```python
from build123d import *
from OCP.BRepFilletAPI import BRepFilletAPI_MakeFillet

# Parameters (mm, degrees)
SKETCH_1_W             = 3
SKETCH_1_H             = 12
SKETCH_1_W_2           = 8
SKETCH_1_H_2           = 3
EXTRUDE_1_DEPTH        = 3
SKETCH_3_R             = 1
CUT_EXTRUDE_1_DEPTH    = 55.203320931
SKETCH_4_W             = 1
SKETCH_4_H             = 7
CUT_EXTRUDE_2_DEPTH    = 55.203320931
SKETCH_6_R             = 1.35
CUT_EXTRUDE_3_DEPTH    = 55.203320931
CUT_EXTRUDE_4_DEPTH    = 55.203320931
CUT_EXTRUDE_6_DEPTH    = 55.203320931
FILLET_1_R             = 2
FILLET_2_R1            = 5
FILLET_2_R2            = 1
FILLET_2_R3            = 2
CUT_EXTRUDE_5602_DEPTH = 55.203320931
FILLET_3_R1            = 1
FILLET_3_R2            = 5


with BuildPart() as part:
    # 草图1 → 凸台-拉伸1 (new body)
    with BuildSketch(Plane(origin=(0, 0, 0), x_dir=(1, 0, 0), z_dir=(0, 1, 0))):
        Polygon((15, 26), (15, 52), (0, 52), (-15, 52), (-15, 46), (0, 0), (7, 0), align=None)
        with Locations((3.5, 9)):
            Rectangle(SKETCH_1_W, SKETCH_1_H, mode=Mode.SUBTRACT)
        with Locations((3.5, 33)):
            Rectangle(SKETCH_1_W, SKETCH_1_H, mode=Mode.SUBTRACT)
        with Locations((-8, 47.5)):
            Rectangle(SKETCH_1_W_2, SKETCH_1_H_2, mode=Mode.SUBTRACT)
        with Locations((8, 47.5)):
            Rectangle(SKETCH_1_W_2, SKETCH_1_H_2, mode=Mode.SUBTRACT)
    extrude(amount=EXTRUDE_1_DEPTH)

    # 草图3 → 切除-拉伸1 (cut, through all)
    with BuildSketch(Plane(origin=(0, 3, 0), x_dir=(1, 0, 0), z_dir=(0, 1, 0))):
        with Locations((5, 4)):
            Circle(SKETCH_3_R)
        with Locations((5, 14)):
            Circle(SKETCH_3_R)
        with Locations((2, 4)):
            Circle(SKETCH_3_R)
        with Locations((2, 14)):
            Circle(SKETCH_3_R)
        with Locations((2, 28)):
            Circle(SKETCH_3_R)
        with Locations((2, 38)):
            Circle(SKETCH_3_R)
        with Locations((5, 28)):
            Circle(SKETCH_3_R)
        with Locations((5, 38)):
            Circle(SKETCH_3_R)
        with Locations((-5, 49)):
            Circle(SKETCH_3_R)
        with Locations((-11, 49)):
            Circle(SKETCH_3_R)
        with Locations((-11, 46)):
            Circle(SKETCH_3_R)
        with Locations((-5, 46)):
            Circle(SKETCH_3_R)
        with Locations((5, 46)):
            Circle(SKETCH_3_R)
        with Locations((11, 46)):
            Circle(SKETCH_3_R)
        with Locations((11, 49)):
            Circle(SKETCH_3_R)
        with Locations((5, 49)):
            Circle(SKETCH_3_R)
    extrude(amount=-CUT_EXTRUDE_1_DEPTH, mode=Mode.SUBTRACT)

    # 草图4 → 切除-拉伸2 (cut, through all)
    with BuildSketch(Plane.XZ):
        with Locations((14.5, -48.5)):
            Rectangle(SKETCH_4_W, SKETCH_4_H)
    extrude(amount=-CUT_EXTRUDE_2_DEPTH, mode=Mode.SUBTRACT)

    # 草图6 → 切除-拉伸3 (cut, through all)
    with BuildSketch(Plane(origin=(0, 3, 0), x_dir=(1, 0, 0), z_dir=(0, 1, 0))):
        with Locations(Location((10, 31, 0), (0, 0, 270))):
            Circle(SKETCH_6_R)
        with Locations(Location((10, 41, 0), (0, 0, 90))):
            Circle(SKETCH_6_R)
    extrude(amount=-CUT_EXTRUDE_3_DEPTH, mode=Mode.SUBTRACT)

    # 草图7 → 切除-拉伸4 (cut, through all)
    with BuildSketch(Plane(origin=(0, 3, 0), x_dir=(1, 0, 0), z_dir=(0, 1, 0))):
        Polygon((-2, 15.810109656), (-10.540181634, 42), (-2, 42), align=None)
    extrude(amount=-CUT_EXTRUDE_4_DEPTH, mode=Mode.SUBTRACT)

    # 草图9 → 切除-拉伸6 (cut, through all)
    with BuildSketch(Plane.XZ):
        Polygon((11.923076923, -16), (9.5, -16), (9.5, -8.125), align=None)
    extrude(amount=-CUT_EXTRUDE_6_DEPTH, mode=Mode.SUBTRACT)

    # 圆角1
    # the kernel refuses this fillet: 2 mm, written as the material it takes off along each edge
    with BuildSketch(Plane(origin=(15, -4.330127019, -45), x_dir=(0, 0, 1), z_dir=(0, 1, 0))) as fillet_1_piece_1:
        with BuildLine():
            CenterArc((1.732050808, -2), FILLET_1_R, 90, 60)
            Line((0, -1), (-0.034641016, -0.98))
            ThreePointArc((-0.034641016, -0.98), (-0.04, -0.5), (-0.04, 0))
            Line((-0.04, 0), (0, 0.04))
            Line((0, 0.04), (1.732050808, 0.04))
            Line((1.732050808, 0.04), (1.732050808, 0))
        make_face()
    extrude(amount=11.660254038, mode=Mode.SUBTRACT)
    with BuildSketch(Plane(origin=(7, -3.692873273, 0), x_dir=(-1, 0, 0), z_dir=(0, 1, 0))) as fillet_1_piece_2:
        with BuildLine():
            CenterArc((FILLET_1_R * 0.738574654518, -FILLET_1_R), FILLET_1_R, 90, 72.897271031)
            Line((-FILLET_1_R * 0.217204354204, -FILLET_1_R * 0.705914151162), (-FILLET_1_R * 0.236319934378, -FILLET_1_R * 0.700032434186))
            Line((-FILLET_1_R * 0.236319934378, -FILLET_1_R * 0.700032434186), (-FILLET_1_R * 0.0147714930904, FILLET_1_R * 0.02))
            Line((-FILLET_1_R * 0.0147714930904, FILLET_1_R * 0.02), (FILLET_1_R * 0.738574654518, FILLET_1_R * 0.02))
            Line((FILLET_1_R * 0.738574654518, FILLET_1_R * 0.02), (FILLET_1_R * 0.738574654518, 0))
        make_face()
    extrude(amount=10.385746545, mode=Mode.SUBTRACT)
    with BuildSketch(Plane(origin=(0, -3.628682784, 0), x_dir=(1, 0, 0), z_dir=(0, 1, 0))) as fillet_1_piece_3:
        with BuildLine():
            CenterArc((FILLET_1_R * 0.725736556818, FILLET_1_R), FILLET_1_R, 198.060471936, 71.939528064)
            Line((-FILLET_1_R * 0.224993282664, FILLET_1_R * 0.689979400169), (-FILLET_1_R * 0.244007879453, FILLET_1_R * 0.683778988172))
            Line((-FILLET_1_R * 0.244007879453, FILLET_1_R * 0.683778988172), (-FILLET_1_R * 0.0145147311364, -FILLET_1_R * 0.02))
            Line((-FILLET_1_R * 0.0145147311364, -FILLET_1_R * 0.02), (FILLET_1_R * 0.725736556818, -FILLET_1_R * 0.02))
            Line((FILLET_1_R * 0.725736556818, -FILLET_1_R * 0.02), (FILLET_1_R * 0.725736556818, 0))
        make_face()
    extrude(amount=10.257365568, mode=Mode.SUBTRACT)
    with BuildSketch(Plane(origin=(-15, -0.794627205, -46), x_dir=(0.31002059983091895, 0, 0.9507298394814782), z_dir=(0, 1, 0))) as fillet_1_piece_4:
        with BuildLine():
            CenterArc((FILLET_1_R * 0.158925440907, FILLET_1_R), FILLET_1_R, 251.939528064, 18.060471936)
            Line((-FILLET_1_R * 0.151095158923, FILLET_1_R * 0.0492701605185), (-FILLET_1_R * 0.15729557092, FILLET_1_R * 0.0302555637289))
            Line((-FILLET_1_R * 0.15729557092, FILLET_1_R * 0.0302555637289), (-FILLET_1_R * 0.00317850881815, -FILLET_1_R * 0.02))
            Line((-FILLET_1_R * 0.00317850881815, -FILLET_1_R * 0.02), (FILLET_1_R * 0.158925440907, -FILLET_1_R * 0.02))
            Line((FILLET_1_R * 0.158925440907, -FILLET_1_R * 0.02), (FILLET_1_R * 0.158925440907, 0))
        make_face()
    extrude(amount=4.589254409, mode=Mode.SUBTRACT)
    with BuildSketch(Plane(origin=(14, -5, -52), x_dir=(-1, 0, 0), z_dir=(0, 1, 0)), Plane(origin=(-15, -5, -52), x_dir=(0, 0, 1), z_dir=(0, 1, 0))) as fillet_1_piece_5:
        with BuildLine():
            CenterArc((FILLET_1_R, FILLET_1_R), FILLET_1_R, 180, 90)
            Line((0, FILLET_1_R), (-FILLET_1_R * 0.02, FILLET_1_R))
            Line((-FILLET_1_R * 0.02, FILLET_1_R), (-FILLET_1_R * 0.02, -FILLET_1_R * 0.02))
            Line((-FILLET_1_R * 0.02, -FILLET_1_R * 0.02), (FILLET_1_R, -FILLET_1_R * 0.02))
            Line((FILLET_1_R, -FILLET_1_R * 0.02), (FILLET_1_R, 0))
        make_face()
    extrude(amount=13, mode=Mode.SUBTRACT)

    # 圆角2: one fillet with a radius per group of edges: ONE call of the kernel's fillet builder (fillet() takes one radius for all edges)
    fillet_2_edges_1 = [part.edges().sort_by_distance(p)[0] for p in [
        (15, 1.5, -26),
    ]]
    fillet_2_edges_2 = [part.edges().sort_by_distance(p)[0] for p in [
        (-10.540181634, 1.5, -42),
        (-2, 1.5, -42),
        (-2, 1.5, -15.810109656),
    ]]
    fillet_2_edges_3 = [part.edges().sort_by_distance(p)[0] for p in [
        (14, 1.5, -45),
    ]]
    fillet_2 = BRepFilletAPI_MakeFillet(part.part.solid().wrapped)
    for e in fillet_2_edges_1:
        fillet_2.Add(FILLET_2_R1, e.wrapped)
    for e in fillet_2_edges_2:
        fillet_2.Add(FILLET_2_R2, e.wrapped)
    for e in fillet_2_edges_3:
        fillet_2.Add(FILLET_2_R3, e.wrapped)
    add(Compound.cast(fillet_2.Shape()), mode=Mode.REPLACE)

    # 草图8 → Cut-Extrude 5602 (cut, through all)
    with BuildSketch(Plane(origin=(0, 3, 0), x_dir=(1, 0, 0), z_dir=(0, 1, 0))):
        with BuildLine():
            Line((9.980196097, 49.02), (6.019803903, 49.02))
            ThreePointArc((6.019803903, 49.02), (4.989999519, 50.019950975), (3.98, 49))
            Line((3.98, 49), (3.98, 46))
            ThreePointArc((3.98, 46), (4.989999519, 44.980049025), (6.019803903, 45.98))
            Line((6.019803903, 45.98), (9.980196097, 45.98))
            ThreePointArc((9.980196097, 45.98), (11.010000481, 44.980049025), (12.02, 46))
            Line((12.02, 46), (12.02, 49))
            ThreePointArc((12.02, 49), (11.010000481, 50.019950975), (9.980196097, 49.02))
        make_face()
        with BuildLine():
            Line((-12.02, 46), (-12.02, 49))
            ThreePointArc((-12.02, 49), (-11.010000481, 50.019950975), (-9.980196097, 49.02))
            Line((-9.980196097, 49.02), (-6.019803903, 49.02))
            ThreePointArc((-6.019803903, 49.02), (-4.989999519, 50.019950975), (-3.98, 49))
            Line((-3.98, 49), (-3.98, 46))
            ThreePointArc((-3.98, 46), (-4.989999519, 44.980049025), (-6.019803903, 45.98))
            Line((-6.019803903, 45.98), (-9.980196097, 45.98))
            ThreePointArc((-9.980196097, 45.98), (-11.010000481, 44.980049025), (-12.02, 46))
        make_face()
        with BuildLine():
            Line((1.98, 36.980196097), (1.98, 29.019803903))
            ThreePointArc((1.98, 29.019803903), (0.980049025, 27.989999519), (2, 26.98))
            Line((2, 26.98), (5, 26.98))
            ThreePointArc((5, 26.98), (6.019950975, 27.989999519), (5.02, 29.019803903))
            Line((5.02, 29.019803903), (5.02, 36.980196097))
            ThreePointArc((5.02, 36.980196097), (6.019950975, 38.010000481), (5, 39.02))
            Line((5, 39.02), (2, 39.02))
            ThreePointArc((2, 39.02), (0.980049025, 38.010000481), (1.98, 36.980196097))
        make_face()
        with BuildLine():
            Line((5, 2.98), (2, 2.98))
            ThreePointArc((2, 2.98), (0.980049025, 3.989999519), (1.98, 5.019803903))
            Line((1.98, 5.019803903), (1.98, 12.980196097))
            ThreePointArc((1.98, 12.980196097), (0.980049025, 14.010000481), (2, 15.02))
            Line((2, 15.02), (5, 15.02))
            ThreePointArc((5, 15.02), (6.019950975, 14.010000481), (5.02, 12.980196097))
            Line((5.02, 12.980196097), (5.02, 5.019803903))
            ThreePointArc((5.02, 5.019803903), (6.019950975, 3.989999519), (5, 2.98))
        make_face()
    extrude(amount=-CUT_EXTRUDE_5602_DEPTH, mode=Mode.SUBTRACT)

    # 圆角3: one fillet with a radius per group of edges: ONE call of the kernel's fillet builder (fillet() takes one radius for all edges)
    fillet_3_edges_1 = [part.edges().sort_by_distance(p)[0] for p in [
        (9.5, 1.5, -16),
        (11.923076923, 1.5, -16),
    ]]
    fillet_3_edges_2 = [part.edges().sort_by_distance(p)[0] for p in [
        (9.5, 1.5, -8.125),
    ]]
    fillet_3 = BRepFilletAPI_MakeFillet(part.part.solid().wrapped)
    for e in fillet_3_edges_1:
        fillet_3.Add(FILLET_3_R1, e.wrapped)
    for e in fillet_3_edges_2:
        fillet_3.Add(FILLET_3_R2, e.wrapped)
    add(Compound.cast(fillet_3.Shape()), mode=Mode.REPLACE)


solid = part.part
```
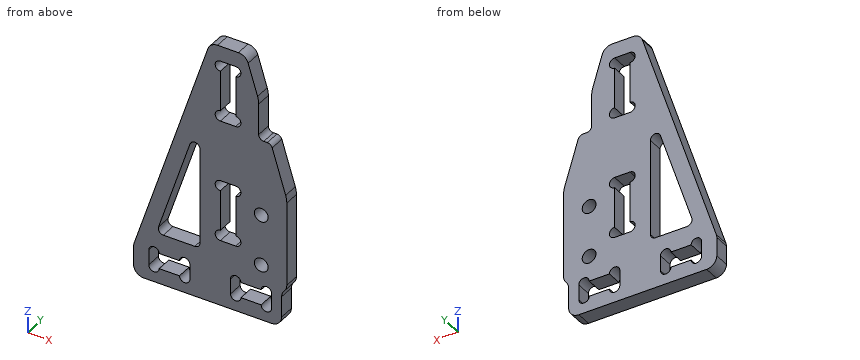
Source: CAD feature listing. Evaluate the final solid. Frame: model axes, mm. Round coordinates to 2 decimals unless told otherwise and drop trailing zeros. Write each loop counter-clockwise with the first axis right and the second up, starting at its lowest first coordinate (ties: lowest second). Pieces come first, ordered by that corner, then holes. Notation, with made-up numbers: M 61,39.25 L 111,39.25 A33 ccw 111,78.25 Z; hole C -31,-9 d2. An arc over 180 degrees is marked long. Answer as a JSON object with one key per item and string values. Group by question number.
(1) Section query C-C on x = -8. Output: boundary loops of the cut face in (y, z).
(2) First-contact query: pin 1 (1 mm diameter, centred on y = 2, z = -11.5, fed in from -X); pin 2 (1.5 mm diameter, centred on y = 2, z = -47.5, fed in from +X); pin 3 (1.5 mm diameter, centred on y = 1, z = -10, fed in from -X); pin 4 (1.5 mm diameter, centred on x = 6.5, z = -34.5, fed in from -Y). Flat tips, straight axial feed; report the tip coordinate or a pass-through.
(3) Ray query, line 1 (Z direction, x = 2.5, y = 0.2); line 2 (Z direction, x = 1.5, y = 2.5); line 3 (X direction, y = 0.6, z = -41). Return the intervals inside material, ascending. Write a range as [from, to].
(4) Section query D-D on z = -14. Output: boundary loops of the cut face in (x, y).
(5) Section query A-A on z = -33.5. Output: boundary loops of the cut face in (x, y).
(6) Section query B-B on x = -2.5. Output: boundary loops of the cut face in (y, z), then the cut area to 3 significant figures.
Computed values:
{
 "1": {"outline": "M 0,-52 L 3,-52 L 3,-49.02 L 0,-49.02 Z; M 0,-45.98 L 3,-45.98 L 3,-42 L 0,-42 Z; M 0,-34.21 L 3,-34.21 L 3,-24.53 L 0,-24.53 Z"},
 "2": {"pin 1": "x = -3.91", "pin 2": "x = 14", "pin 3": "x = -3.51", "pin 4": "y = 0"},
 "3": {"line 1": "[-52, -39.02], [-26.98, -15.02], [-2.98, 0]", "line 2": "[-52, -38.89], [-37.11, -28.89], [-27.11, -14.89], [-13.11, -4.89], [-3.11, 0]", "line 3": "[-13.37, -10.16], [-2, 8.65], [11.35, 15]"},
 "4": {"outline": "M -4.57,0 L 0.98,0 L 0.98,3 L -4.57,3 Z; M 6.02,0 L 9.5,0 L 9.5,3 L 6.02,3 Z"},
 "5": {"outline": "M -10.92,0 L -7.77,0 L -7.77,3 L -10.92,3 Z; M -2,0 L 1.98,0 L 1.98,3 L -2,3 Z; M 5.02,0 L 15,0 L 15,3 L 5.02,3 Z"},
 "6": {"outline": "M 0,-52 L 3,-52 L 3,-41.87 L 0,-41.87 Z; M 0,-21.24 L 3,-21.24 L 3,-7.67 L 0,-7.67 Z", "area": "71.1 mm^2"}
}
